For this review, take the finished solid that the model builds, in its own axes (mm). Round coordinates to 2 decimals unless told otherwise and drop trailing zeros. Loops run counter-clockwise (first coordinate to the right, second up) from the corner with the lowest first, then second, coordinate; pieces in that order, holes last.
1. To check wall thickness, follow line 1 along X through (y, z) = (1.9, 0); line 2 along Z through (x, y) = (335, 0.4); line 3 along Z through (x, y) = (-41.5, 0.95). State the ranges of each line that lie inside material, in increasing order.
2. Consider section A-A on x = 210. State the section outline as (y, z) points (3 decimals).
3. Clearance check with flat-ended pins moving along their axes: pin 1 Ø5.5 at (x, z) = (-25.4, -355.6) entering from +Y; pin 2 Ø1 at (x, y) = (319.5, 2) entering from +Z; pin 3 Ø1.5 at (x, y) = (223, 2.5) entering from -Z. State where each tip first meets the part, or that it passes through.
4. Consider section B-B on z = 108. State the section outline as (x, y) points (3 decimals).
5. Consider section C-C on y = 0.7. State how many separate pieces and enclosed holes the cut face has, then the cut area to 3 significant figures.
from build123d import *

# Parameters (mm, degrees)
SKETCH1_R           = 2.413
BOSS_EXTRUDE2_DEPTH = 3.175
FILLET2_R           = 3.175
SKETCH2_R           = 1.63195
CUT_EXTRUDE1_DEPTH  = 5.08
SKETCH3_R           = 4.445
CUT_EXTRUDE2_DEPTH  = 5.08
SKETCH8_R           = 3.048
CUT_EXTRUDE3_DEPTH  = 16.256


with BuildPart() as part:
    # Sketch1 → Boss-Extrude2 (new body)
    with BuildSketch(Plane(origin=(0, 0, 0), x_dir=(1, 0, 0), z_dir=(0, 1, 0))):
        Polygon((368.3, 139.7), (368.3, 190.500003027), (342.9, 190.500003027), (342.9, 184.150003027), (285.749996671, 184.150003027), (171.449996973, 298.45), (171.449996973, 368.3), (-171.450003027, 368.3), (-171.450003027, 298.45), (-298.45, 171.45), (-368.3, 171.45), (-368.3, -171.45), (-298.450006054, -171.45), (-171.450003027, -298.45), (-171.450003027, -368.3), (171.449996973, -368.3), (171.449996973, -298.45), (285.750002724, -184.149996973), (342.9, -184.149996973), (342.9, -190.499996973), (368.3, -190.499996973), (368.3, -139.7), (241.3, -139.7), (241.3, 139.7), align=None)
        with Locations(Location((-152.400003027, -355.6, 0), (0, 0, 270))):
            Circle(SKETCH1_R, mode=Mode.SUBTRACT)
        with Locations(Location((-76.200003027, -355.6, 0), (0, 0, 270))):
            Circle(SKETCH1_R, mode=Mode.SUBTRACT)
        with Locations(Location((-3.027e-06, -355.6, 0), (0, 0, 270))):
            Circle(SKETCH1_R, mode=Mode.SUBTRACT)
        with Locations(Location((-355.6, -152.4, 0), (0, 0, 270))):
            Circle(SKETCH1_R, mode=Mode.SUBTRACT)
        with Locations(Location((-355.6, -76.2, 0), (0, 0, 270))):
            Circle(SKETCH1_R, mode=Mode.SUBTRACT)
        with Locations(Location((76.199996973, -355.6, 0), (0, 0, 270))):
            Circle(SKETCH1_R, mode=Mode.SUBTRACT)
        with Locations(Location((50.8, -279.399996973, 0), (0, 0, 270))):
            Circle(SKETCH1_R, mode=Mode.SUBTRACT)
        with Locations(Location((76.2, -279.399996973, 0), (0, 0, 270))):
            Circle(SKETCH1_R, mode=Mode.SUBTRACT)
        with Locations(Location((152.399996973, -355.6, 0), (0, 0, 270))):
            Circle(SKETCH1_R, mode=Mode.SUBTRACT)
        with Locations(Location((101.6, -279.399996973, 0), (0, 0, 270))):
            Circle(SKETCH1_R, mode=Mode.SUBTRACT)
        with Locations(Location((127, -279.399996973, 0), (0, 0, 270))):
            Circle(SKETCH1_R, mode=Mode.SUBTRACT)
        with Locations(Location((152.4, -279.399996973, 0), (0, 0, 270))):
            Circle(SKETCH1_R, mode=Mode.SUBTRACT)
        with Locations(Location((50.8, -152.399996973, 0), (0, 0, 270))):
            Circle(SKETCH1_R, mode=Mode.SUBTRACT)
        with Locations(Location((152.4, -152.399996973, 0), (0, 0, 270))):
            Circle(SKETCH1_R, mode=Mode.SUBTRACT)
        with Locations(Location((254, -152.399996973, 0), (0, 0, 270))):
            Circle(SKETCH1_R, mode=Mode.SUBTRACT)
        with Locations(Location((355.6, -152.399996973, 0), (0, 0, 270))):
            Circle(SKETCH1_R, mode=Mode.SUBTRACT)
        with Locations(Location((-355.6, 0, 0), (0, 0, 270))):
            Circle(SKETCH1_R, mode=Mode.SUBTRACT)
        with Locations(Location((-355.6, 76.2, 0), (0, 0, 270))):
            Circle(SKETCH1_R, mode=Mode.SUBTRACT)
        with Locations(Location((-355.6, 152.4, 0), (0, 0, 270))):
            Circle(SKETCH1_R, mode=Mode.SUBTRACT)
        with Locations(Location((-152.4, 355.6, 0), (0, 0, 270))):
            Circle(SKETCH1_R, mode=Mode.SUBTRACT)
        with Locations(Location((-76.2, 355.6, 0), (0, 0, 270))):
            Circle(SKETCH1_R, mode=Mode.SUBTRACT)
        with Locations(Location((0, 355.6, 0), (0, 0, 270))):
            Circle(SKETCH1_R, mode=Mode.SUBTRACT)
        with Locations(Location((50.8, 152.400003027, 0), (0, 0, 270))):
            Circle(SKETCH1_R, mode=Mode.SUBTRACT)
        with Locations(Location((152.4, 152.400003027, 0), (0, 0, 270))):
            Circle(SKETCH1_R, mode=Mode.SUBTRACT)
        with Locations(Location((254, 152.400003027, 0), (0, 0, 270))):
            Circle(SKETCH1_R, mode=Mode.SUBTRACT)
        with Locations(Location((355.6, 152.400003027, 0), (0, 0, 270))):
            Circle(SKETCH1_R, mode=Mode.SUBTRACT)
        with Locations(Location((50.8, 279.400003027, 0), (0, 0, 270))):
            Circle(SKETCH1_R, mode=Mode.SUBTRACT)
        with Locations(Location((76.2, 279.400003027, 0), (0, 0, 270))):
            Circle(SKETCH1_R, mode=Mode.SUBTRACT)
        with Locations(Location((76.2, 355.6, 0), (0, 0, 270))):
            Circle(SKETCH1_R, mode=Mode.SUBTRACT)
        with Locations(Location((101.6, 279.400003027, 0), (0, 0, 270))):
            Circle(SKETCH1_R, mode=Mode.SUBTRACT)
        with Locations(Location((127, 279.400003027, 0), (0, 0, 270))):
            Circle(SKETCH1_R, mode=Mode.SUBTRACT)
        with Locations(Location((152.4, 279.400003027, 0), (0, 0, 270))):
            Circle(SKETCH1_R, mode=Mode.SUBTRACT)
        with Locations(Location((152.4, 355.6, 0), (0, 0, 270))):
            Circle(SKETCH1_R, mode=Mode.SUBTRACT)
        with Locations(Location((355.6, 177.800003027, 0), (0, 0, 270))):
            Circle(SKETCH1_R, mode=Mode.SUBTRACT)
        with Locations(Location((355.6, -177.799996973, 0), (0, 0, 270))):
            Circle(SKETCH1_R, mode=Mode.SUBTRACT)
    extrude(amount=BOSS_EXTRUDE2_DEPTH)

    # Fillet2
    fillet2_edges = [part.edges().sort_by_distance(p)[0] for p in [
        (171.449996973, 1.5875, 298.45),
        (-171.450003027, 1.5875, 368.3),
        (-171.450003027, 1.5875, 298.45),
        (-298.450006054, 1.5875, 171.45),
        (-368.3, 1.5875, 171.45),
        (-368.3, 1.5875, -171.45),
        (-298.45, 1.5875, -171.45),
        (-171.450003027, 1.5875, -298.45),
        (-171.450003027, 1.5875, -368.3),
        (171.449996973, 1.5875, -368.3),
        (171.449996973, 1.5875, -298.45),
        (171.449996973, 1.5875, 368.3),
        (241.3, 1.5875, 139.7),
        (368.3, 1.5875, 139.7),
        (285.750002724, 1.5875, 184.149996973),
        (285.749996671, 1.5875, -184.150003027),
        (368.3, 1.5875, -139.7),
        (241.3, 1.5875, -139.7),
        (342.9, 1.5875, 190.499996973),
        (342.9, 1.5875, 184.149996973),
        (342.9, 1.5875, -184.150003027),
        (342.9, 1.5875, -190.500003027),
        (368.3, 1.5875, -190.500003027),
        (368.3, 1.5875, 190.499996973),
    ]]
    fillet(fillet2_edges, radius=FILLET2_R - 0.0001)  # a hair under: the kernel refuses the full size

    # Sketch2 → Cut-Extrude1 (cut)
    with BuildSketch(Plane(origin=(0, 3.175, 0), x_dir=(1, 0, 0), z_dir=(0, 1, 0))):
        with Locations(Location((14.478, 1.778, 0), (0, 0, 270))):
            Circle(SKETCH2_R)
        with Locations(Location((-14.478, -27.178, 0), (0, 0, 270))):
            Circle(SKETCH2_R)
    extrude(amount=-CUT_EXTRUDE1_DEPTH, mode=Mode.SUBTRACT)

    # Sketch3 → Cut-Extrude2 (cut)
    with BuildSketch(Plane.XZ):
        with Locations(Location((-25.4, -355.6, 0), (0, 0, 270))):
            Circle(SKETCH3_R)
        with Locations(Location((-38.1, -355.6, 0), (0, 0, 270))):
            Circle(SKETCH3_R)
        with Locations(Location((-50.8, -355.6, 0), (0, 0, 270))):
            Circle(SKETCH3_R)
        with Locations(Location((-50.8, 355.6, 0), (0, 0, 90))):
            Circle(SKETCH3_R)
        with Locations(Location((-38.1, 355.6, 0), (0, 0, 90))):
            Circle(SKETCH3_R)
        with Locations(Location((-25.4, 355.6, 0), (0, 0, 90))):
            Circle(SKETCH3_R)
    extrude(amount=-CUT_EXTRUDE2_DEPTH, mode=Mode.SUBTRACT)

    # Sketch8 → Cut-Extrude3 (cut)
    with BuildSketch(Plane(origin=(0, 3.175, 0), x_dir=(1, 0, 0), z_dir=(0, 1, 0))):
        with Locations(Location((-38.1, -171.45, 0), (0, 0, 270))):
            Circle(SKETCH8_R)
        with Locations(Location((-38.1, 171.45, 0), (0, 0, 270))):
            Circle(SKETCH8_R)
        with Locations(Location((-38.1, 0, 0), (0, 0, 270))):
            Circle(SKETCH8_R)
    extrude(amount=-CUT_EXTRUDE3_DEPTH, mode=Mode.SUBTRACT)


solid = part.part
Resolved:
1. line 1: x = -368.3 to -358.01, -353.19 to -41.15, -35.05 to 241.3
1. line 2: z = -184.15 to -139.7, 139.7 to 184.15
1. line 3: z = -368.3 to -358.46, -352.74 to 352.74, 358.46 to 368.3
2. outline: (0, -259.9) - (3.175, -259.9) - (3.175, 259.9) - (0, 259.9) - close
3. pin 1: passes through
3. pin 2: stops at z = 184.15
3. pin 3: stops at z = -247.65
4. outline: (-368.3, 0) - (241.3, 0) - (241.3, 3.175) - (-368.3, 3.175) - close
5. separate pieces: 1
5. enclosed holes: 46
5. area: 385,000 mm2
